Build history of the part. All positions in model axes, mm. A direction names the side the tool comes from. Round coordinates to 2 decimals unless told otherwise and drop trailing zeros. Answer in a Markdown table with one row per item. Add a question column.
from build123d import *

# Parameters (mm, degrees)
BOSS_EXTRUDE1_DEPTH = 6.62
CUT_EXTRUDE1_REACH  = 8.62
CUT_EXTRUDE2_REACH  = 8.62
SKETCH3_R           = 1.6
SKETCH4_R           = 2.75
CUT_EXTRUDE3_DEPTH  = 3.2
SKETCH6_R           = 9.95
CUT_EXTRUDE4_DEPTH  = 10
SKETCH7_R           = 12.5
CUT_EXTRUDE5_DEPTH  = 3
CUT_EXTRUDE9_REACH  = 8.62
SKETCH10_R          = 1.600000003
SKETCH11_R          = 2.750000001
CUT_EXTRUDE10_DEPTH = 3
SKETCH12_W          = 31
SKETCH12_H          = 20.5
CUT_EXTRUDE11_DEPTH = 3
CUT_EXTRUDE12_REACH = 8.62
SKETCH13_R          = 1.6
SKETCH14_R          = 2.75
CUT_EXTRUDE13_DEPTH = 1.5
CUT_EXTRUDE14_REACH = 8.62
SKETCH15_R          = 1.1


with BuildPart() as part:
    # Sketch1 → Boss-Extrude1 (new body)
    with BuildSketch(Plane.XY):
        with BuildLine():
            Line((-53.15, -20.367507575), (-350.15, -20.367507575))
            ThreePointArc((-350.15, -20.367507575), (-370.15, -0.367507575), (-350.15, 19.632492425))
            Line((-350.15, 19.632492425), (-53.15, 19.632492425))
            ThreePointArc((-53.15, 19.632492425), (-33.15, -0.367507575), (-53.15, -20.367507575))
        make_face()
    extrude(amount=BOSS_EXTRUDE1_DEPTH)

    # Sketch2 → Cut-Extrude1 (cut, up to next)
    with BuildSketch(Plane(origin=(0, 0, 0), x_dir=(-1, 0, 0), z_dir=(0, 0, -1)), mode=Mode.PRIVATE) as cut_extrude1_sk1:
        with BuildLine():
            Line((53.15, 7.282492425), (63.133045479, 7.282492425))
            ThreePointArc((63.133045479, 7.282492425), (63.830991164, 5.41363036), (64.33147081, 3.482492425))
            Line((64.33147081, 3.482492425), (77.35, 3.482492425))
            ThreePointArc((77.35, 3.482492425), (81.2, -0.367507575), (77.35, -4.217507575))
            Line((77.35, -4.217507575), (64.33147081, -4.217507575))
            ThreePointArc((64.33147081, -4.217507575), (63.830991164, -6.14864551), (63.133045479, -8.017507575))
            Line((63.133045479, -8.017507575), (53.15, -8.017507575))
            ThreePointArc((53.15, -8.017507575), (45.5, -0.367507575), (53.15, 7.282492425))
        make_face()
    cut_extrude1_tool1 = extrude(cut_extrude1_sk1.sketch, amount=-CUT_EXTRUDE1_REACH, mode=Mode.PRIVATE) & part.part
    add(cut_extrude1_tool1.solids().sort_by_distance((-60.965388, -0.367508, 0))[0], mode=Mode.SUBTRACT)

    # Sketch3 → Cut-Extrude2 (cut, up to next)
    with BuildSketch(Plane(origin=(0, 0, 0), x_dir=(-1, 0, 0), z_dir=(0, 0, -1)), mode=Mode.PRIVATE) as cut_extrude2_sk1:
        with Locations((77.715530374, -12.367507575)):
            Circle(SKETCH3_R)
    cut_extrude2_tool1 = extrude(cut_extrude2_sk1.sketch, amount=-CUT_EXTRUDE2_REACH, mode=Mode.PRIVATE) & part.part
    add(cut_extrude2_tool1.solids().sort_by_distance((-77.71553, -12.367508, 0))[0], mode=Mode.SUBTRACT)
    # Sketch3 → Cut-Extrude2 (cut, up to next)
    with BuildSketch(Plane(origin=(0, 0, 0), x_dir=(-1, 0, 0), z_dir=(0, 0, -1)), mode=Mode.PRIVATE) as cut_extrude2_sk2:
        with Locations((77.715530374, 11.632492425)):
            Circle(SKETCH3_R)
    cut_extrude2_tool2 = extrude(cut_extrude2_sk2.sketch, amount=-CUT_EXTRUDE2_REACH, mode=Mode.PRIVATE) & part.part
    add(cut_extrude2_tool2.solids().sort_by_distance((-77.71553, 11.632492, 0))[0], mode=Mode.SUBTRACT)
    # Sketch3 → Cut-Extrude2 (cut, up to next)
    with BuildSketch(Plane(origin=(0, 0, 0), x_dir=(-1, 0, 0), z_dir=(0, 0, -1)), mode=Mode.PRIVATE) as cut_extrude2_sk3:
        with Locations((56.965530374, 11.632492425)):
            Circle(SKETCH3_R)
    cut_extrude2_tool3 = extrude(cut_extrude2_sk3.sketch, amount=-CUT_EXTRUDE2_REACH, mode=Mode.PRIVATE) & part.part
    add(cut_extrude2_tool3.solids().sort_by_distance((-56.96553, 11.632492, 0))[0], mode=Mode.SUBTRACT)
    # Sketch3 → Cut-Extrude2 (cut, up to next)
    with BuildSketch(Plane(origin=(0, 0, 0), x_dir=(-1, 0, 0), z_dir=(0, 0, -1)), mode=Mode.PRIVATE) as cut_extrude2_sk4:
        with Locations((56.965530374, -12.367507575)):
            Circle(SKETCH3_R)
    cut_extrude2_tool4 = extrude(cut_extrude2_sk4.sketch, amount=-CUT_EXTRUDE2_REACH, mode=Mode.PRIVATE) & part.part
    add(cut_extrude2_tool4.solids().sort_by_distance((-56.96553, -12.367508, 0))[0], mode=Mode.SUBTRACT)

    # Sketch4 → Cut-Extrude3 (cut)
    with BuildSketch(Plane(origin=(0, 0, 0), x_dir=(-1, 0, 0), z_dir=(0, 0, -1))):
        with Locations((56.965530374, 11.632492425)):
            Circle(SKETCH4_R)
        with Locations((77.715530374, 11.632492425)):
            Circle(SKETCH4_R)
        with Locations((77.715530374, -12.367507575)):
            Circle(SKETCH4_R)
        with Locations((56.965530374, -12.367507575)):
            Circle(SKETCH4_R)
    extrude(amount=-CUT_EXTRUDE3_DEPTH, mode=Mode.SUBTRACT)

    # Sketch6 → Cut-Extrude4 (cut)
    with BuildSketch(Plane.XY.offset(6.62)):
        with Locations((-350.15, -0.367507575)):
            Circle(SKETCH6_R)
    extrude(amount=-CUT_EXTRUDE4_DEPTH, mode=Mode.SUBTRACT)

    # Sketch7 → Cut-Extrude5 (cut)
    with BuildSketch(Plane(origin=(0, 0, 0), x_dir=(-1, 0, 0), z_dir=(0, 0, -1))):
        with Locations((350.15, -0.367507575)):
            Circle(SKETCH7_R)
    extrude(amount=-CUT_EXTRUDE5_DEPTH, mode=Mode.SUBTRACT)

    # Sketch10 → Cut-Extrude9 (cut, up to next)
    with BuildSketch(Plane.XY.offset(6.62), mode=Mode.PRIVATE) as cut_extrude9_sk1:
        with Locations((-207.590530375, -8.367507581)):
            Circle(SKETCH10_R)
    cut_extrude9_tool1 = extrude(cut_extrude9_sk1.sketch, amount=-CUT_EXTRUDE9_REACH, mode=Mode.PRIVATE) & part.part
    add(cut_extrude9_tool1.solids().sort_by_distance((-207.59053, -8.367508, 6.62))[0], mode=Mode.SUBTRACT)
    # Sketch10 → Cut-Extrude9 (cut, up to next)
    with BuildSketch(Plane.XY.offset(6.62), mode=Mode.PRIVATE) as cut_extrude9_sk2:
        with Locations((-207.590530375, 7.632492419)):
            Circle(SKETCH10_R)
    cut_extrude9_tool2 = extrude(cut_extrude9_sk2.sketch, amount=-CUT_EXTRUDE9_REACH, mode=Mode.PRIVATE) & part.part
    add(cut_extrude9_tool2.solids().sort_by_distance((-207.59053, 7.632492, 6.62))[0], mode=Mode.SUBTRACT)
    # Sketch10 → Cut-Extrude9 (cut, up to next)
    with BuildSketch(Plane.XY.offset(6.62), mode=Mode.PRIVATE) as cut_extrude9_sk3:
        with Locations((-167.917908126, -8.367507581)):
            Circle(SKETCH10_R)
    cut_extrude9_tool3 = extrude(cut_extrude9_sk3.sketch, amount=-CUT_EXTRUDE9_REACH, mode=Mode.PRIVATE) & part.part
    add(cut_extrude9_tool3.solids().sort_by_distance((-167.917908, -8.367508, 6.62))[0], mode=Mode.SUBTRACT)
    # Sketch10 → Cut-Extrude9 (cut, up to next)
    with BuildSketch(Plane.XY.offset(6.62), mode=Mode.PRIVATE) as cut_extrude9_sk4:
        with Locations((-167.917908126, 7.632492419)):
            Circle(SKETCH10_R)
    cut_extrude9_tool4 = extrude(cut_extrude9_sk4.sketch, amount=-CUT_EXTRUDE9_REACH, mode=Mode.PRIVATE) & part.part
    add(cut_extrude9_tool4.solids().sort_by_distance((-167.917908, 7.632492, 6.62))[0], mode=Mode.SUBTRACT)

    # Sketch11 → Cut-Extrude10 (cut)
    with BuildSketch(Plane(origin=(0, 0, 0), x_dir=(-1, 0, 0), z_dir=(0, 0, -1))):
        with Locations((207.590530375, 7.632492419)):
            Circle(SKETCH11_R)
        with Locations((207.590530375, -8.367507581)):
            Circle(SKETCH11_R)
        with Locations((167.917908126, 7.632492419)):
            Circle(SKETCH11_R)
        with Locations((167.917908126, -8.367507581)):
            Circle(SKETCH11_R)
    extrude(amount=-CUT_EXTRUDE10_DEPTH, mode=Mode.SUBTRACT)

    # Sketch12 → Cut-Extrude11 (cut)
    with BuildSketch(Plane.XY.offset(6.62)):
        with Locations((-304.957095584, 9.382492425)):
            Rectangle(SKETCH12_W, SKETCH12_H)
    extrude(amount=-CUT_EXTRUDE11_DEPTH, mode=Mode.SUBTRACT)

    # Sketch13 → Cut-Extrude12 (cut, up to next)
    with BuildSketch(Plane.XY.offset(6.62), mode=Mode.PRIVATE) as cut_extrude12_sk1:
        with Locations((-311.957095584, 7.632492425)):
            Circle(SKETCH13_R)
    cut_extrude12_tool1 = extrude(cut_extrude12_sk1.sketch, amount=-CUT_EXTRUDE12_REACH, mode=Mode.PRIVATE) & part.part
    add(cut_extrude12_tool1.solids().sort_by_distance((-311.957096, 7.632492, 6.62))[0], mode=Mode.SUBTRACT)
    # Sketch13 → Cut-Extrude12 (cut, up to next)
    with BuildSketch(Plane.XY.offset(6.62), mode=Mode.PRIVATE) as cut_extrude12_sk2:
        with Locations((-297.957095584, 7.632492425)):
            Circle(SKETCH13_R)
    cut_extrude12_tool2 = extrude(cut_extrude12_sk2.sketch, amount=-CUT_EXTRUDE12_REACH, mode=Mode.PRIVATE) & part.part
    add(cut_extrude12_tool2.solids().sort_by_distance((-297.957096, 7.632492, 6.62))[0], mode=Mode.SUBTRACT)

    # Sketch14 → Cut-Extrude13 (cut)
    with BuildSketch(Plane(origin=(0, 0, 0), x_dir=(-1, 0, 0), z_dir=(0, 0, -1))):
        with Locations((311.957095584, 7.632492425)):
            Circle(SKETCH14_R)
        with Locations((297.957095584, 7.632492425)):
            Circle(SKETCH14_R)
    extrude(amount=-CUT_EXTRUDE13_DEPTH, mode=Mode.SUBTRACT)

    # Sketch15 → Cut-Extrude14 (cut, up to next)
    with BuildSketch(Plane.XY.offset(6.62), mode=Mode.PRIVATE) as cut_extrude14_sk1:
        with Locations((-151.644507933, -18.367507575)):
            Circle(SKETCH15_R)
    cut_extrude14_tool1 = extrude(cut_extrude14_sk1.sketch, amount=-CUT_EXTRUDE14_REACH, mode=Mode.PRIVATE) & part.part
    add(cut_extrude14_tool1.solids().sort_by_distance((-151.644508, -18.367508, 6.62))[0], mode=Mode.SUBTRACT)
    # Sketch15 → Cut-Extrude14 (cut, up to next)
    with BuildSketch(Plane.XY.offset(6.62), mode=Mode.PRIVATE) as cut_extrude14_sk2:
        with Locations((-92.280362099, -18.367507575)):
            Circle(SKETCH15_R)
    cut_extrude14_tool2 = extrude(cut_extrude14_sk2.sketch, amount=-CUT_EXTRUDE14_REACH, mode=Mode.PRIVATE) & part.part
    add(cut_extrude14_tool2.solids().sort_by_distance((-92.280362, -18.367508, 6.62))[0], mode=Mode.SUBTRACT)
    # Sketch15 → Cut-Extrude14 (cut, up to next)
    with BuildSketch(Plane.XY.offset(6.62), mode=Mode.PRIVATE) as cut_extrude14_sk3:
        with Locations((-151.644507933, 17.632492425)):
            Circle(SKETCH15_R)
    cut_extrude14_tool3 = extrude(cut_extrude14_sk3.sketch, amount=-CUT_EXTRUDE14_REACH, mode=Mode.PRIVATE) & part.part
    add(cut_extrude14_tool3.solids().sort_by_distance((-151.644508, 17.632492, 6.62))[0], mode=Mode.SUBTRACT)
    # Sketch15 → Cut-Extrude14 (cut, up to next)
    with BuildSketch(Plane.XY.offset(6.62), mode=Mode.PRIVATE) as cut_extrude14_sk4:
        with Locations((-92.280362099, 17.632492425)):
            Circle(SKETCH15_R)
    cut_extrude14_tool4 = extrude(cut_extrude14_sk4.sketch, amount=-CUT_EXTRUDE14_REACH, mode=Mode.PRIVATE) & part.part
    add(cut_extrude14_tool4.solids().sort_by_distance((-92.280362, 17.632492, 6.62))[0], mode=Mode.SUBTRACT)
    # Sketch15 → Cut-Extrude14 (cut, up to next)
    with BuildSketch(Plane.XY.offset(6.62), mode=Mode.PRIVATE) as cut_extrude14_sk5:
        with Locations((-222.491552839, 17.632492425)):
            Circle(SKETCH15_R)
    cut_extrude14_tool5 = extrude(cut_extrude14_sk5.sketch, amount=-CUT_EXTRUDE14_REACH, mode=Mode.PRIVATE) & part.part
    add(cut_extrude14_tool5.solids().sort_by_distance((-222.491553, 17.632492, 6.62))[0], mode=Mode.SUBTRACT)
    # Sketch15 → Cut-Extrude14 (cut, up to next)
    with BuildSketch(Plane.XY.offset(6.62), mode=Mode.PRIVATE) as cut_extrude14_sk6:
        with Locations((-283.750452743, 17.632492425)):
            Circle(SKETCH15_R)
    cut_extrude14_tool6 = extrude(cut_extrude14_sk6.sketch, amount=-CUT_EXTRUDE14_REACH, mode=Mode.PRIVATE) & part.part
    add(cut_extrude14_tool6.solids().sort_by_distance((-283.750453, 17.632492, 6.62))[0], mode=Mode.SUBTRACT)


solid = part.part
(1) Drop flat-ended pins along their axis: P1, Ø1, axis at y = -3, z = 4.5, coming from the +X side; P2, Ø1.5, axis at y = 8.5, z = 4.5, coming from the -X side; P3, Ø4, axis at x = -311.96, y = 7.63, coming from the +Z side. Give the stop position or say it passes through.
(2) Probe line 1 along X through (y, z) = (-17.5, 4.5); line 2 along X through (y, z) = (0.5, 1.75); line 3 along Y through (x, z) = (-350.15, 5). List the from-to ranges inside material, lowest first.
(3) Mould opens along Y. For faces 3 (the face through (-81.2, -0.3, 3.3)), 4 (the face through (-370.145, -0.807, 3.264)) say: pulls with the +Y half, pulls with the -Y half, needs draft (parallel to the pull), parting line crosses it, or undercut.
(4) Saw through at A-A (z = 5.25). Count the separate pieces of the cut face and the enclosed holes in it, plus the area to 3 significant figures.
(5) Which spindle directions (+Z, -Z, +X, -X, +Y, -Y) get a long thin tool onto all of the face, cutting with end or side? Do faces 1 (the face through (-169, -10, 3)), 2 (the face through (-45.5, -0.5, 3.3)). Say none if no direction does.
Answer sheet:
| question | item | result |
|---|---|---|
| 1 | P1 | stops at x = -33.26 |
| 1 | P2 | stops at x = -368.43 |
| 1 | P3 | stops at z = 3.62 |
| 2 | line 1 | x = -360.47 to -152.32, -150.97 to -92.96, -91.6 to -42.83 |
| 2 | line 2 | x = -370.13 to -362.62, -337.68 to -81.1, -45.55 to -33.17 |
| 2 | line 3 | y = -20.37 to -10.32, 9.58 to 19.63 |
| 3 | face 3 | undercut |
| 3 | face 4 | parting line crosses it |
| 4 | separate pieces | 1 |
| 4 | enclosed holes | 16 |
| 4 | area | 11,700 mm² |
| 5 | face 1 | -Z |
| 5 | face 2 | +Z, -Z |
